from build123d import *

# Parameters (mm, degrees)
ESBO_O1_R                = 2
RESSALTO_EXTRUS_O1_DEPTH = 5


with BuildPart() as part:
    # Esboço1 → Ressalto-extrusão1 (new body)
    # profile 1 of 2: a face of its own
    with BuildSketch(Plane(origin=(0, 0, 0), x_dir=(1, 0, 0), z_dir=(0, 1, 0))):
        with BuildLine():
            Line((9.016735984, -20.218643644), (16.087803796, -27.289711456))
            ThreePointArc((16.087803796, -27.289711456), (21.087803796, -27.289711456), (21.087803796, -22.289711456))
            Line((21.087803796, -22.289711456), (14.016735984, -15.218643644))
            Line((14.016735984, -15.218643644), (14.016735984, 48.781356356))
            ThreePointArc((14.016735984, 48.781356356), (13.138056327, 50.902676699), (11.016735984, 51.781356356))
            Line((11.016735984, 51.781356356), (-75.983264016, 51.781356356))
            Line((-75.983264016, 51.781356356), (-80.983264016, 46.781356356))
            Line((-80.983264016, 46.781356356), (-80.983264016, -17.218643644))
            ThreePointArc((-80.983264016, -17.218643644), (-80.10458436, -19.339963988), (-77.983264016, -20.218643644))
            Line((-77.983264016, -20.218643644), (9.016735984, -20.218643644))
        make_face()
        with Locations(Location((16.30226989, -22.50417755, 0), (0, 0, 270))):
            Circle(ESBO_O1_R, mode=Mode.SUBTRACT)
    # profile 2 of 2: a face of its own
    with BuildSketch(Plane(origin=(0, 0, 0), x_dir=(1, 0, 0), z_dir=(0, 1, 0))):
        with BuildLine():
            Line((-75.983264016, 51.781356356), (-83.054331828, 58.852424167))
            ThreePointArc((-83.054331828, 58.852424167), (-88.054331828, 58.852424167), (-88.054331828, 53.852424167))
            Line((-88.054331828, 53.852424167), (-80.983264016, 46.781356356))
            Line((-80.983264016, 46.781356356), (-75.983264016, 51.781356356))
        make_face()
        with Locations(Location((-83.268797922, 54.066890262, 0), (0, 0, 270))):
            Circle(ESBO_O1_R, mode=Mode.SUBTRACT)
    extrude(amount=RESSALTO_EXTRUS_O1_DEPTH)


solid = part.part
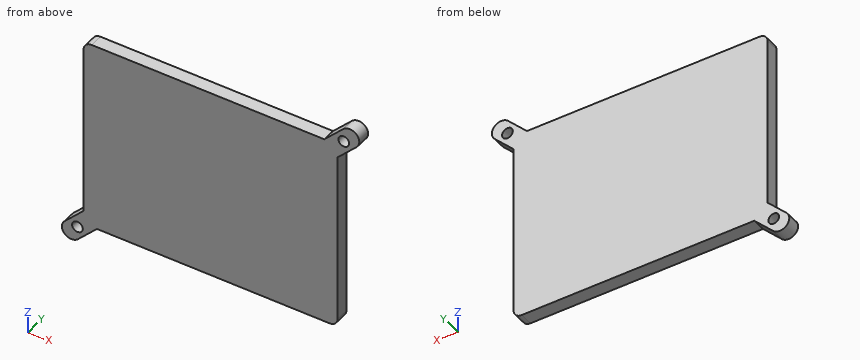
The model under review builds one solid part; all positions refer to its coordinate system, in mm. Give positions to 0.01 mm unless a question says otherwise; leave off trailing zeros. Write each loop counter-clockwise with the first axis right and the second up, starting at its lowest first coordinate (ties: lowest second). Pieces come first, ordered by that corner, then holes. Notation, with made-up numbers: M 31.25,-3.75 L 69.25,-3.75 A33 ccw 69.25,24.25 Z; hole C -0.75,47.5 d2. An arc over 180 degrees is marked long. One line per question, with ' | ' between items. Start each with the question number.
Item 1: We need section C-C on z = -22. Write out the cut boundary in (x, y), plus the area to 3 significant figures.
Item 2: We need section A-A on x = -32. Write out the cut boundary in (y, z), plus the area to 3 significant figures.
Item 3: Wall thickness on line 1 (X direction, y = 2.05, z = -2.5); line 2 (Z direction, x = 2.5, y = 3.9); line 3 (X direction, y = 1.4, z = -47.5): over which ranges is each line inside the solid? List them lowest first. Write a range as from..to.
Item 4: For pin 1 (2.5 mm diameter, centred on x = 16.3, z = 22.5, fed in from +Y); pin 2 (2 mm diameter, centred on x = -9, y = 2, fed in from -Z); pin 3 (3 mm diameter, centred on y = 0.5, z = -35, fed in from -X); pin 4 (3 mm diameter, centred on x = -17, y = 2, fed in from +Z), all flat-tipped, find the tip position at first contact; note any pin that passes through.
Item 5: We need section B-B on y = 2.3. Write out the cut boundary in (x, z), plus the area to 3 significant figures.
Results found:
1) outline: M -80.98,0 L 14.02,0 L 14.02,5 L -80.98,5 Z | area: 475 mm2
2) outline: M 0,-51.78 L 5,-51.78 L 5,20.22 L 0,20.22 Z | area: 360 mm2
3) line 1: x = -80.98..14.02 | line 2: z = -51.78..20.22 | line 3: x = -81.7..14.02
4) pin 1: passes through | pin 2: stops at z = -51.78 | pin 3: stops at x = -80.98 | pin 4: stops at z = 20.22
5) outline: M -88.05,-53.85 A3.54 ccw -83.05,-58.85 L -75.98,-51.78 L 11.02,-51.78 A3 ccw 14.02,-48.78 L 14.02,15.22 L 21.09,22.29 A3.54 ccw 16.09,27.29 L 9.02,20.22 L -77.98,20.22 A3 ccw -80.98,17.22 L -80.98,-46.78 Z; hole C -83.27,-54.07 d4; hole C 16.3,22.5 d4 | area: 6,970 mm2
